Source: CAD feature listing. Evaluate the final solid. Frame: model axes, mm. A direction names the side the tool comes from. Coordinates: 2 decimals unless noted, no trailing zeros. Write each loop counter-clockwise with the first axis right and the second up, starting at its lowest first coordinate (ties: lowest second). Pieces come first, ordered by that corner, then holes. Notation, with made-up numbers: (-16, 51.25) -> (-6, 51.25) arc R20 cw to (-6, 84.25) -> close; hole circle Ø7 at (-11.75, 53). An arc over 180 degrees is marked (long way). One line per item, written item: value. Start each with the question number.
1. Access query for faces 4 (the cylindrical face through (-52.783, 10.554, 1.972)), 5 (the cylindrical face through (-70.398, 11.414, 8.93)). Directions: +Z, -Z, +X, -X, +Y, -Y. A direction counts if a zero-diameter tool reaches every point of the face in a straight line with its end or side. Return the directions, or none.
2. Section query C-C, the plane z = 3.5. Output: boundary loops of the cut face in (x, y).
3. Section query D-D, the plane x = -64. Output: boundary loops of the cut face in (y, z).
4. Mould query, pull axis Y, two halves, no side actions, for faces 1 (the flat face through (-73, 5.664, 2)), 2 (the flat face through (-73, 11, 0)), 3 (the cylindrical face through (-86.438, 12.772, 1.972)). Classes: released by +Y, released by -Y, zero draft, split by the parting line, or undercut.
5. First-contact query: P1, Ø4, axis at y = 9, z = 9.5, coming from the -X side; P2, Ø3, axis at x = -76, y = 8.5, coming from the +Z side; P3, Ø1, axis at x = -75, z = 11, coming from the +Y side. Flat tips, straight axial feed; report the tip coordinate or a pass-through.
6. Section query B-B, the plane y = 10. Output: boundary loops of the cut face in (x, z), and give its area (3 significant figures).
7. Line query: line 1 (X direction, y = 10.5, z = 3.75); line 2 (Z direction, x = -68.5, y = 7.25); line 3 (Y direction, x = -57.5, z = 2). Output: solid intervals per line, ascending.
8. Section query A-A, the plane x = -86.5. Output: boundary loops of the cut face in (y, z).
from build123d import *

# Parameters (mm, degrees)
SKETCH1_R           = 2.5
BOSS_EXTRUDE1_DEPTH = 4
SKETCH2_R           = 2.5
BOSS_EXTRUDE2_DEPTH = 10


with BuildPart() as part:
    # Sketch1 → Boss-Extrude1 (new body)
    with BuildSketch(Plane.XY):
        with BuildLine():
            Line((-57.782253853, 15.663533632), (-87.782253853, 15.663533632))
            ThreePointArc((-87.782253853, 15.663533632), (-92.782253853, 10.663533632), (-87.782253853, 5.663533632))
            Line((-87.782253853, 5.663533632), (-57.782253853, 5.663533632))
            ThreePointArc((-57.782253853, 5.663533632), (-52.782253853, 10.663533632), (-57.782253853, 15.663533632))
        make_face()
        with Locations((-57.782253853, 10.663533632)):
            Circle(SKETCH1_R, mode=Mode.SUBTRACT)
        with Locations((-87.782253853, 10.663533632)):
            Circle(SKETCH1_R, mode=Mode.SUBTRACT)
    extrude(amount=BOSS_EXTRUDE1_DEPTH)

    # Sketch2 → Boss-Extrude2 (add)
    with BuildSketch(Plane.XY.offset(4)):
        with Locations((-72.782253853, 10.663533632)):
            Circle(SKETCH2_R)
    extrude(amount=BOSS_EXTRUDE2_DEPTH)


solid = part.part
Computed values:
1. face 4: +Z, -Z, +X
1. face 5: +Z
2. outline: (-87.78, 5.66) -> (-57.78, 5.66) arc R5 ccw to (-57.78, 15.66) -> (-87.78, 15.66) arc R5 ccw to start; hole circle Ø5 at (-87.78, 10.66); hole circle Ø5 at (-57.78, 10.66)
3. outline: (5.66, 0) -> (15.66, 0) -> (15.66, 4) -> (5.66, 4) -> close
4. face 1: released by -Y
4. face 2: zero draft
4. face 3: undercut
5. P1: stops at x = -75.28
5. P2: stops at z = 14
5. P3: stops at y = 12.48
6. outline: (-92.74, 0) -> (-90.19, 0) -> (-90.19, 4) -> (-92.74, 4) -> close; (-85.37, 0) -> (-60.19, 0) -> (-60.19, 4) -> (-70.37, 4) -> (-70.37, 14) -> (-75.19, 14) -> (-75.19, 4) -> (-85.37, 4) -> close; (-55.37, 0) -> (-52.83, 0) -> (-52.83, 4) -> (-55.37, 4) -> close
6. area: 169 mm²
7. line 1: x = -92.78 to -90.28, -85.29 to -60.28, -55.29 to -52.78
7. line 2: z = 0 to 4
7. line 3: y = 5.67 to 8.18, 13.15 to 15.66
8. outline: (5.66, 0) -> (8.52, 0) -> (8.52, 4) -> (5.66, 4) -> close; (12.81, 0) -> (15.66, 0) -> (15.66, 4) -> (12.81, 4) -> close
